Check sheet for the modelled part. Datum: model origin and axes. Units: mm. Face numbers are marked on the shaded views. Give positions to 0.01 mm unless a question says otherwise; leave off trailing zeros. Write each loop counter-clockwise with the first axis right and the second up, starting at its lowest first coordinate (ties: lowest second). Pieces come first, ordered by that corner, then holes. Notation, with made-up numbers: M 75,-37.5 L 107,-37.5 A13 cw 107,-21.5 Z; hole C -28.5,33 d1. An arc over 180 degrees is marked long. Write item = value, one per line. Start each with the question number.
1) Gauge pin test, flat ends, axial feed: pin 1 (3 mm diameter, centred on x = 11.5, y = -5, fed in from +Z); pin 2 (1.5 mm diameter, centred on x = -2.5, z = -10.5, fed in from +Y); pin 3 (12 mm diameter, centred on x = 11, z = -2, fed in from -Y); pin 4 (3 mm diameter, centred on x = 0, z = 0, fed in from -Y). Record the tip position at first contact, or that the pin passes through.
2) Scan lines: L1, parallel to Z at x = 0, y = -3.8; L2, parallel to Y at x = 6, z = -15; L3, parallel to X at y = -0.5, z = -6.5. Record each from-to range of solid material in increasing order.
3) Sectioned sample at A-A, the plane y = -7. Record the cut outline in (x, z).
4) Sectioned sample at B-B, the plane y = -4. Record the cut outline in (x, z).
5) Draft check along X on the marked faces 1 and 2. Enter one of: pulls with the +X half, pulls with the -X half, needs draft (parallel to the pull), parting line crosses it, or undercut.
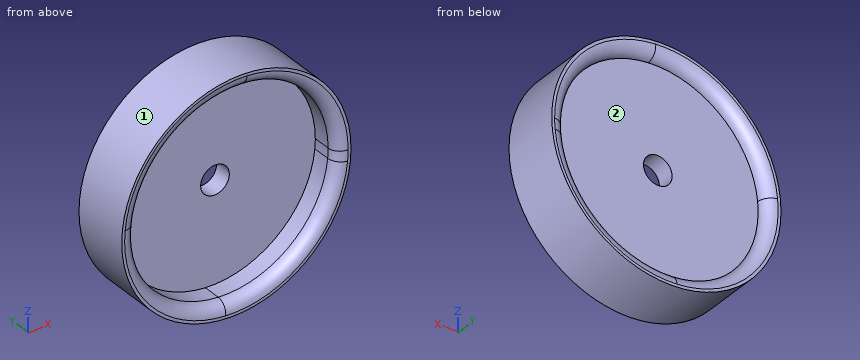
from build123d import *

# Parameters (mm, degrees)
F0_R     = 20
F1_DEPTH = 10
F2_START = 2
F2_DEPTH = 3
F3_R     = 1.99999
F4_D     = 5


# Not quite as in the source:
# - a fillet or chamfer is up to 0.001 mm smaller than in the source, because OpenCascade refuses the exact size


with BuildPart() as f1:
    # F0 (on Front) → F1 (new body)
    with BuildSketch(Plane.XZ):
        Circle(F0_R)
        with BuildLine():
            ThreePointArc((1.6759297538, 17.4195654211), (12.9533542122, 11.766928854), (17.5, 0))
            ThreePointArc((17.5, 0), (17.4798797889, -0.8389294162), (17.4195654211, -1.6759297538))
            ThreePointArc((17.4195654211, -1.6759297538), (11.1324315409, -13.5025541283), (-1.6759297538, -17.4195654211))
            ThreePointArc((-1.6759297538, -17.4195654211), (-13.5025541283, -11.1324315409), (-17.4195654211, 1.6759297538))
            ThreePointArc((-17.4195654211, 1.6759297538), (-11.1324315409, 13.5025541283), (1.6759297538, 17.4195654211))
        make_face(mode=Mode.SUBTRACT)
    extrude(amount=F1_DEPTH)

    # F0 (on Front) → F2 (join)
    with BuildSketch(Plane.XZ.offset(F2_START)):
        with BuildLine():
            Line((0, 0), (1.6759297538, 17.4195654211))
            ThreePointArc((1.6759297538, 17.4195654211), (-11.1324315409, 13.5025541283), (-17.4195654211, 1.6759297538))
            Line((-17.4195654211, 1.6759297538), (0, 0))
        make_face()
        with BuildLine():
            ThreePointArc((-1.6759297538, -17.4195654211), (11.1324315409, -13.5025541283), (17.4195654211, -1.6759297538))
            Line((17.4195654211, -1.6759297538), (0, 0))
            Line((0, 0), (-1.6759297538, -17.4195654211))
        make_face()
        with BuildLine():
            Line((0, 0), (-17.4195654211, 1.6759297538))
            ThreePointArc((-17.4195654211, 1.6759297538), (-13.5025541283, -11.1324315409), (-1.6759297538, -17.4195654211))
            Line((-1.6759297538, -17.4195654211), (0, 0))
        make_face()
        with BuildLine():
            ThreePointArc((17.4195654211, -1.6759297538), (17.4798797889, -0.8389294162), (17.5, 0))
            ThreePointArc((17.5, 0), (12.9533542122, 11.766928854), (1.6759297538, 17.4195654211))
            Line((1.6759297538, 17.4195654211), (0, 0))
            Line((0, 0), (17.4195654211, -1.6759297538))
        make_face()
    extrude(amount=F2_DEPTH)

    # F3 (radius 2 in the source; OpenCascade refuses exactly that, so slightly less here)
    f3_edges = [f1.edges().sort_by_distance(p)[0] for p in [
        (-17.5, -10, 0),
        (-17.5, 0, 0),
    ]]
    fillet(f3_edges, radius=F3_R)

    # F4 (through all)
    with Locations(Plane(origin=(0, 0, 0), x_dir=(1, 0, 0), z_dir=(0, 1, 0))):
        with Locations((0, 0)):
            Hole(F4_D / 2)


solid = f1.part
Data:
q1.pin_1 = 17.32
q1.pin_2 = -2
q1.pin_3 = -5
q1.pin_4 = through
q2.L1 = -20 to -2.5, 2.5 to 20
q2.L2 = -5 to -2
q2.L3 = -18.91 to -16.98, 16.98 to 18.91
q3.outline = C 0,0 d40; hole C 0,0 d35
q4.outline = C 0,0 d40; hole C 0,0 d5
q5.face_1 = parting line crosses it
q5.face_2 = undercut
